Geometry: final body of the model. Coordinates: model frame, mm. A direction names the side the tool comes from. Give positions to 0.01 mm unless a question says otherwise; leave off trailing zeros. Loops run counter-clockwise (first coordinate to the right, second up) from the corner with the lowest first, then second, coordinate; pieces in that order, holes last.
1. First-contact query: P1, Ø3, axis at x = -4.5, y = 1, coming from the -Z side; P2, Ø6, axis at x = -4.5, y = -5, coming from the -Z side; P3, Ø2, axis at x = 4.5, z = 88, coming from the +Y side. Flat tips, straight axial feed; report the tip coordinate or a pass-through.
2. Access query for faces 1 (the face through (-2, 6, 148)), 2 (the face through (-1.73, -7.81, 72.96)), 3 (the face through (5.723, -1.802, -3.451)). Directions: +Z, -Z, +X, -X, +Y, -Y. A direction counts if a zero-diameter tool reaches every point of the face in a straight line with its end or side. Return the directions, or none.
3. Material intervals for line 1 along Z through (x, y) = (-5.75, 3.25); line 2 along Z through (x, y) = (4, -4); line 3 along Y through (x, z) = (0.25, 47.5), sorted ascending.
4. Section C-C, the plane z = 91.5. Output: boundary loops of the cut face in (x, y).
from build123d import *

# Parameters (mm, degrees)
SKETCH1_R           = 8
BOSS_EXTRUDE1_DEPTH = 148
SKETCH6_R           = 6
BOSS_EXTRUDE2_DEPTH = 5
SKETCH7_R           = 6
BOSS_EXTRUDE3_DEPTH = 2
SKETCH8_R           = 5
BOSS_EXTRUDE4_DEPTH = 10
SKETCH9_R           = 4
BOSS_EXTRUDE5_DEPTH = 10
CHAMFER1_SIZE       = 1
CHAMFER2_SIZE       = 1
BOSS_EXTRUDE6_START = 5
SKETCH10_R          = 6
BOSS_EXTRUDE6_DEPTH = 5
BOSS_EXTRUDE7_START = 2
SKETCH11_R          = 6
BOSS_EXTRUDE7_DEPTH = 2
BOSS_EXTRUDE8_START = 10
SKETCH12_R          = 5
BOSS_EXTRUDE8_DEPTH = 10
CHAMFER3_SIZE       = 1


with BuildPart() as part:
    # Sketch1 → Boss-Extrude1 (new body)
    with BuildSketch(Plane.XY):
        Circle(SKETCH1_R)
    extrude(amount=BOSS_EXTRUDE1_DEPTH)

    # Sketch6 → Boss-Extrude2 (add)
    with BuildSketch(Plane(origin=(0, 0, 0), x_dir=(-1, 0, 0), z_dir=(0, 0, -1))):
        with Locations(Location((0, 0, 0), (0, 0, 180))):
            Circle(SKETCH6_R)
    extrude(amount=BOSS_EXTRUDE2_DEPTH)

    # Sketch7 → Boss-Extrude3 (add)
    with BuildSketch(Plane(origin=(0, 0, -5), x_dir=(-1, 0, 0), z_dir=(0, 0, -1))):
        with Locations(Location((0, 0, 0), (0, 0, 180))):
            Circle(SKETCH7_R)
    extrude(amount=BOSS_EXTRUDE3_DEPTH)

    # Sketch8 → Boss-Extrude4 (add)
    with BuildSketch(Plane(origin=(0, 0, -7), x_dir=(-1, 0, 0), z_dir=(0, 0, -1))):
        Circle(SKETCH8_R)
    extrude(amount=BOSS_EXTRUDE4_DEPTH)

    # Sketch9 → Boss-Extrude5 (add)
    with BuildSketch(Plane(origin=(0, 0, -17), x_dir=(-1, 0, 0), z_dir=(0, 0, -1))):
        Circle(SKETCH9_R)
    extrude(amount=BOSS_EXTRUDE5_DEPTH)

    # Chamfer1
    chamfer1_edges = [part.edges().sort_by_distance(p)[0] for p in [
        (5, 0, -17),
    ]]
    chamfer(chamfer1_edges, length=CHAMFER1_SIZE - 0.0001)  # a hair under: the kernel refuses the full size

    # Chamfer2
    chamfer2_edges = [part.edges().sort_by_distance(p)[0] for p in [
        (4, 0, -27),
    ]]
    chamfer(chamfer2_edges, length=CHAMFER2_SIZE)

    # Sketch10 → Boss-Extrude6 (add)
    with BuildSketch(Plane.XY.offset(148).offset(BOSS_EXTRUDE6_START)):
        Circle(SKETCH10_R)
    extrude(amount=-BOSS_EXTRUDE6_DEPTH)

    # Sketch11 → Boss-Extrude7 (add)
    with BuildSketch(Plane.XY.offset(153).offset(BOSS_EXTRUDE7_START)):
        Circle(SKETCH11_R)
    extrude(amount=-BOSS_EXTRUDE7_DEPTH)

    # Sketch12 → Boss-Extrude8 (add)
    with BuildSketch(Plane.XY.offset(155).offset(BOSS_EXTRUDE8_START)):
        with Locations(Location((0, 0, 0), (0, 0, 180))):
            Circle(SKETCH12_R)
    extrude(amount=-BOSS_EXTRUDE8_DEPTH)

    # Chamfer3
    chamfer3_edges = [part.edges().sort_by_distance(p)[0] for p in [
        (5, 0, 165),
    ]]
    chamfer(chamfer3_edges, length=CHAMFER3_SIZE)


solid = part.part
Answers below:
1. P1: stops at z = -26.89
1. P2: stops at z = -26.27
1. P3: stops at y = 7.19
2. face 1: +Z
2. face 2: +Z, -Z
2. face 3: -Z
3. line 1: z = 0 to 148
3. line 2: z = -7 to 155
3. line 3: y = -8 to 8
4. outline: circle Ø16 at (0, 0)
